Here's the drawing with two shaded views (mm, measured from the low corner). I have some questions. Give positions to 0.01 mm unless a question says otherwise; leave off trailing zeros. Write each loop counter-clockwise with the first axis right and the second up, starting at its lowest first coordinate (ties: lowest second). Pieces come first, ordered by that corner, then holes. Notation, with made-up numbers: M 20,2 L 44,2 A32 cw 44,33 Z; hole C 84.25,-25.5 d8. An arc over 180 degrees is marked long. Use one line per item in the form item = value. Start each with the question number.
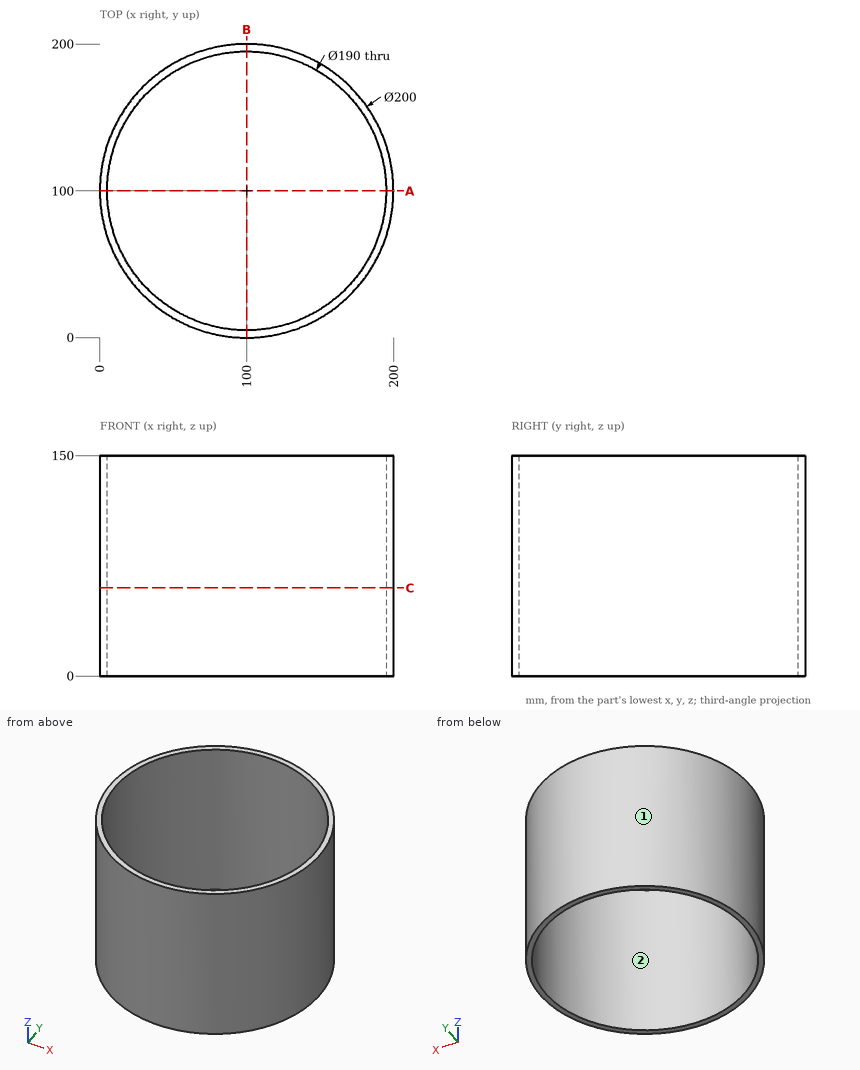
1) Thinking about a two-plate mould opening in X: for the marked faces 1 and 2, which applies, released by +X, released by -X, zero draft, split by the parting line, or undercut?
2) Suppose I cut it at C-C, the plane z = 60. List the corners of the cut face in (x, y) for me.
3) Suppose I cut it at A-A, the plane y = 100. List the corners of the cut face in (x, z) for me, and give its area (3 significant figures).
4) Please list where these lines run through material, in increasing order: line 1 (Y direction, x = 100, z = 49.5); line 2 (X direction, y = 28, z = 32); line 3 (Y direction, x = 64.5, z = 104).
5) Will these pins go through, and if not, where does the flat tip stop? P1, Ø10, axis at y = 94.5, z = 121.5, coming from the +X side; P2, Ø4, axis at x = 157, z = 77.5, coming from the -Y side; P3, Ø1.5, axis at y = 53.5, z = 68, coming from the -X side.
Checks:
q1.face_1 = split by the parting line
q1.face_2 = undercut
q2.outline = C 100,100 d200; hole C 100,100 d190
q3.outline = M 0,0 L 5,0 L 5,150 L 0,150 Z; M 195,0 L 200,0 L 200,150 L 195,150 Z
q3.area = 1,500 mm^2
q4.line_1 = 0 to 5, 195 to 200
q4.line_2 = 30.6 to 38.02, 161.98 to 169.4
q4.line_3 = 6.51 to 11.88, 188.12 to 193.49
q5.P1 = 200
q5.P2 = 16.48
q5.P3 = 11.08
